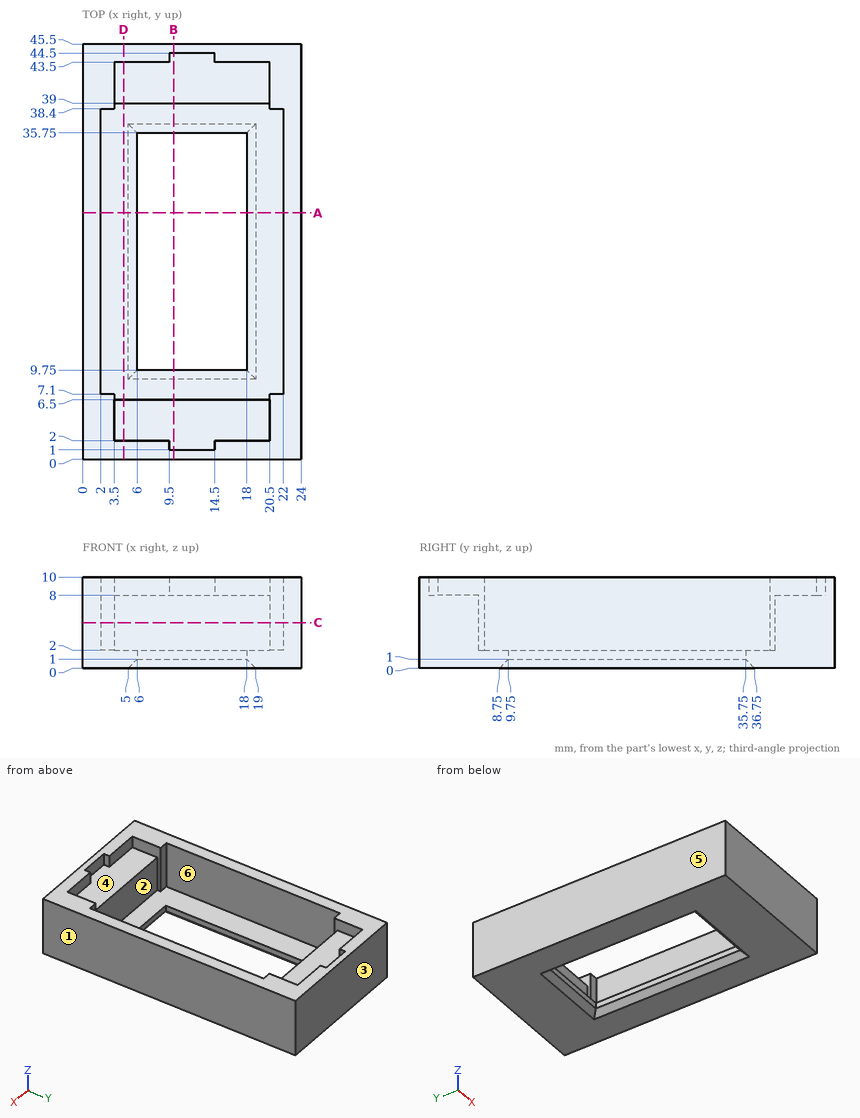
The figure shows three views and two pictorial views of one solid part (mm, origin at its lowest corner). Answer the questions. A direction names the side the tool comes from. Round coordinates to 2 decimals unless told otherwise and drop trailing zeros. Loops run counter-clockwise (first coordinate to the right, second up) from the corner with the lowest first, then second, coordinate; pieces in that order, holes last. Notation, with made-up numbers: M 4,-16.75 L 25,-16.75 A22 cw 25,-3.75 Z; hole C 35,-9.75 d7. An arc over 180 degrees is marked long. Use CSV: the item, a comma, the result in double quotes.
Q1. The mould has two halves that part along Y. Classify the marked faces 1, 2, 3 and 4: pulls with the +Y half, pulls with the -Y half, needs draft (parallel to the pull), parting line crosses it, or undercut.
Determined:
face 1,"needs draft"
face 2,"undercut"
face 3,"pulls with the +Y half"
face 4,"undercut"
Q2. A tool of negligible diameter and unlimited length cuts with its end or side. For the marked faces 5 and 6, from which of +Z, -Z, +X, -X, +Y, -Y can it reach the whole face along a straight path? Write none if from no direction.
Determined:
face 5,"+Z, -Z, -X, +Y, -Y"
face 6,"+Z"
Q3. Consider L1, parallel to X at y = 20, z = 5.25; L2, parallel to X at y = 31.5, z = 1; L3, parallel to Y at x = 5, z = 3.75. Determine where each line is inside the solid, lowest interval first.
Determined:
L1,"0 to 2, 22 to 24"
L2,"0 to 6, 18 to 24"
L3,"0 to 6.5, 39 to 45.5"
Q4. Section C-C, the plane z = 5 is taken. Determine the outline of the cut face in (x, y), then the cut area to 3 significant figures.
Determined:
outline,"M 0,0 L 24,0 L 24,45.5 L 0,45.5 Z; hole M 2,7.1 L 3.5,7.1 L 3.5,6.5 L 20.5,6.5 L 20.5,7.1 L 22,7.1 L 22,38.4 L 20.5,38.4 L 20.5,39 L 3.5,39 L 3.5,38.4 L 2,38.4 Z"
area,"446 mm2"
Q5. Section D-D, the plane x = 4.5 is taken. Determine the outline of the cut face in (y, z), then the cut area to 3 significant figures.
Determined:
outline,"M 0,0 L 45.5,0 L 45.5,10 L 43.5,10 L 43.5,8 L 39,8 L 39,2 L 6.5,2 L 6.5,8 L 2,8 L 2,10 L 0,10 Z"
area,"177 mm2"
Q6. Section A-A, the plane y = 27 is taken. Determine the outline of the cut face in (x, z), then the cut area to 3 significant figures.
Determined:
outline,"M 0,0 L 5,0 L 6,1 L 6,2 L 2,2 L 2,10 L 0,10 Z; M 18,1 L 19,0 L 24,0 L 24,10 L 22,10 L 22,2 L 18,2 Z"
area,"55.0 mm2"
Q7. Each of these flat-tipped pins is pushed along its axis until it touches: pin 1 (5 mm diameter, centred on x = 19, y = 16.5, fed in from +Z); pin 2 (6 mm diameter, centred on x = 12.5, y = 41, fed in from +Z). Where does it stop, or does it pass through?
Determined:
pin 1,"z = 2"
pin 2,"z = 8"
Q8. Section B-B, the plane x = 10 is taken. Determine the outline of the cut face in (y, z), then the cut area to 3 significant figures.
Determined:
outline,"M 0,0 L 8.75,0 L 9.75,1 L 9.75,2 L 6.5,2 L 6.5,8 L 1,8 L 1,10 L 0,10 Z; M 35.75,1 L 36.75,0 L 45.5,0 L 45.5,10 L 44.5,10 L 44.5,8 L 39,8 L 39,2 L 35.75,2 Z"
area,"120 mm2"
